Check sheet for the modelled part. Datum: model origin and axes. Units: mm. Coordinates: 2 decimals unless noted, no trailing zeros. Write each loop counter-clockwise with the first axis right and the second up, starting at its lowest first coordinate (ties: lowest second). Pieces come first, ordered by that corner, then holes. Notation, with made-up numbers: (44, 84) -> (80, 84) arc R32 cw to (80, 114) -> close; hole circle Ø6 at (59.25, -32.75). An arc over 180 degrees is marked (long way). One line per item, written item: value. Start each with the question number.
1) Scan lines: line 1 along Z through (x, y) = (85, 1.5); line 2 along Z through (x, y) = (10, 2.25); line 3 along X through (y, z) = (2.5, -86). Record each from-to range of solid material in increasing order. Write a range as [from, to].
2) Draft check along Z on faces 1 (the flat face through (37, 5, -49)), 2 (the cylindrical face through (85.806, 2.465, -78.265)), 3 (the flat face through (47, 2, -96)), 4 (the cylindrical face through (86.43, 2.46, -19.45)). Enter one of: +Z half, -Z half, draft (parallel to the pull), parting line (faces both ways), or undercut.
3) Sectioned sample at C-C on z = -77. Enter the section's corners in (x, y), plus the area to 3 significant figures.
4) Sectioned sample at B-B on z = -48. Enter the section's corners in (x, y), plus the area to 3 significant figures.
5) Sectioned sample at A-A on x = 10. Enter the section's corners in (y, z).
```python
from build123d import *

# Parameters (mm, degrees)
SKETCH1_W           = 96
SKETCH1_H           = 96
SKETCH1_R           = 1.5
BOSS_EXTRUDE1_DEPTH = 5
SKETCH2_R           = 4.7625
CUT_EXTRUDE1_DEPTH  = 6


with BuildPart() as part:
    # Sketch1 → Boss-Extrude1 (new body)
    with BuildSketch(Plane(origin=(0, 0, 0), x_dir=(1, 0, 0), z_dir=(0, 1, 0))):
        with Locations((48, 48)):
            Rectangle(SKETCH1_W, SKETCH1_H)
        with Locations((10, 10)):
            Circle(SKETCH1_R, mode=Mode.SUBTRACT)
        with Locations((85, 19)):
            Circle(SKETCH1_R, mode=Mode.SUBTRACT)
        with Locations((85, 77)):
            Circle(SKETCH1_R, mode=Mode.SUBTRACT)
        with Locations((10, 86)):
            Circle(SKETCH1_R, mode=Mode.SUBTRACT)
    extrude(amount=BOSS_EXTRUDE1_DEPTH)

    # Sketch2 → Cut-Extrude1 (cut, through all)
    with BuildSketch(Plane(origin=(0, 5, 0), x_dir=(1, 0, 0), z_dir=(0, 1, 0))):
        with Locations((48, 48)):
            Circle(SKETCH2_R)
    extrude(amount=-CUT_EXTRUDE1_DEPTH, mode=Mode.SUBTRACT)


solid = part.part
```
Answers:
1. line 1: z = [-96, -78.5], [-75.5, -20.5], [-17.5, 0]
1. line 2: z = [-96, -87.5], [-84.5, -11.5], [-8.5, 0]
1. line 3: x = [0, 8.5], [11.5, 96]
2. face 1: draft
2. face 2: undercut
2. face 3: -Z half
2. face 4: undercut
3. outline: (0, 0) -> (83.5, 0) -> (83.5, 5) -> (0, 5) -> close; (86.5, 0) -> (96, 0) -> (96, 5) -> (86.5, 5) -> close
3. area: 465 mm2
4. outline: (0, 0) -> (43.24, 0) -> (43.24, 5) -> (0, 5) -> close; (52.76, 0) -> (96, 0) -> (96, 5) -> (52.76, 5) -> close
4. area: 432 mm2
5. outline: (0, -96) -> (5, -96) -> (5, -87.5) -> (0, -87.5) -> close; (0, -84.5) -> (5, -84.5) -> (5, -11.5) -> (0, -11.5) -> close; (0, -8.5) -> (5, -8.5) -> (5, 0) -> (0, 0) -> close
